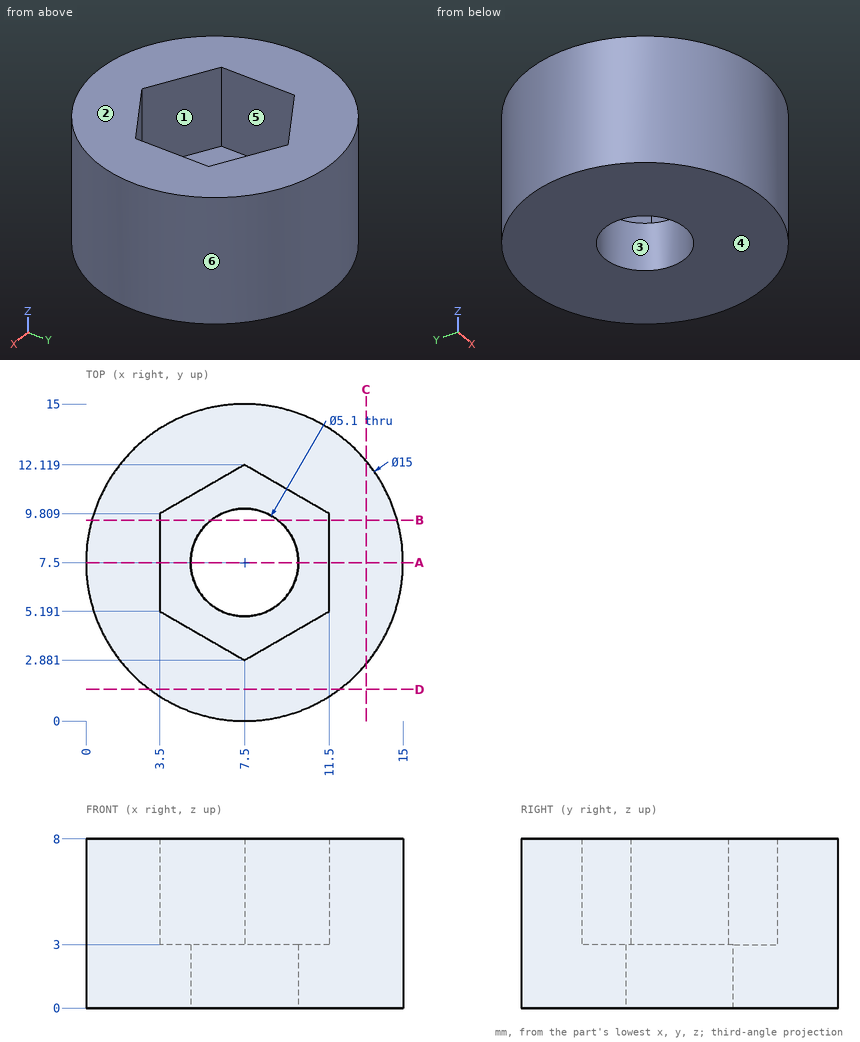
Job drawing, mm, ordinate dimensions from the low corner. One solid piece. A direction names the side the tool comes from. Coordinates: 2 decimals unless noted, no trailing zeros. Order: outer loops, then holes, each group sorted by start corner. A loop starts at its lowest first (then second) coordinate and runs counter-clockwise, first axis right, second up. Notation, with made-up numbers: (73, 65) - (121, 65) arc R16 ccw to (121, 92) - close; hole circle Ø10 at (-21, 31). An arc over 180 degrees is marked (long way). Return JSON: item names as keys, results as strings. Group by question number.
1) Tool access for the marked faces 1 and 2: list every direction of +Z, -Z, +X, -X, +Y, -Y with a clear straight run to the whole face (end or side of a thin tool).
2) Saw through at A-A, the plane y = 7.5. Write the cut outline in (x, z), plus the area to 3 significant figures.
3) Saw through at B-B, the plane y = 9.5. Write the cut outline in (x, z).
4) Mould opens along X. For the marked faces 3, 4, 5 and 6 say: released by +X, released by -X, zero draft, split by the parting line, or undercut.
5) Probe line 1 (X direction, y = 7.5, z = 0.8); line 2 (Y direction, x = 8, z = 1.5); line 3 (X direction, y = 7, z = 6.25). List the from-to ranges inside material, lowest first. Write a range as from..to.
6) Saw through at C-C, the plane x = 13.25. Write the cut outline in (y, z) (1 decimal).
7) Saw through at D-D, the plane y = 1.5. Write the cut outline in (x, z).
8) Flat gauge pins, fed straight in: P1, Ø2, axis at x = 12, z = 6, coming from the +Y side; P2, Ø4, axis at y = 4.5, z = 1.5, coming from the -X side; P3, Ø4, axis at x = 1.5, z = 5, coming from the +Y side (1 decimal). Where does each tip first touch, or does it go through?
Values found:
{
 "1": {"face 1": "+Z", "face 2": "+Z, +X, -X, +Y, -Y"},
 "2": {"outline": "(0, 0) - (4.95, 0) - (4.95, 3) - (3.5, 3) - (3.5, 8) - (0, 8) - close; (10.05, 0) - (15, 0) - (15, 8) - (11.5, 8) - (11.5, 3) - (10.05, 3) - close", "area": "64.7 mm²"},
 "3": {"outline": "(0.27, 0) - (5.92, 0) - (5.92, 3) - (3.5, 3) - (3.5, 8) - (0.27, 8) - close; (9.08, 0) - (14.73, 0) - (14.73, 8) - (11.5, 8) - (11.5, 3) - (9.08, 3) - close"},
 "4": {"face 3": "undercut", "face 4": "zero draft", "face 5": "undercut", "face 6": "split by the parting line"},
 "5": {"line 1": "x = 0..4.95, 10.05..15", "line 2": "y = 0.02..5, 10..14.98", "line 3": "x = 0.02..3.5, 11.5..14.98"},
 "6": {"outline": "(2.7, 0) - (12.3, 0) - (12.3, 8) - (2.7, 8) - close"},
 "7": {"outline": "(3, 0) - (12, 0) - (12, 8) - (3, 8) - close"},
 "8": {"P1": "stops at y = 14.13", "P2": "stops at x = 0.07", "P3": "stops at y = 13.8"}
}
